Autodesk Inventor part; units mm, degrees
ref_plane "YZ Plane" through (0, 0, 0) normal (1, 0, 0) x (0, 1, 0)
ref_plane "XZ Plane" through (0, 0, 0) normal (0, 1, 0) x (-1, 0, 0)
ref_plane "XY Plane" through (0, 0, 0) normal (0, 0, 1) x (1, 0, 0)
sketch "Sketch1" plane through (0, 0, 0) normal (0, 0, 1) x (1, 0, 0)
  line L0 (-15.5, -9) -> (15.5, -9)
  line L1 (15.5, -9) -> (15.5, 9)
  line L2 (15.5, 9) -> (-15.5, 9)
  line L3 (-15.5, 9) -> (-15.5, -9)
  line L4 (-15.5, -9) -> (15.5, 9) construction
  line L5 (15.5, -9) -> (-15.5, 9) construction
  point P0 (0, 0)
  dimension "d0" = 31
  dimension "d1" = 18
extrude "Extrusion1" add sketch "Sketch1" along normal blind 12.5
sketch "Sketch4" plane through (-15.5, -9, 0) normal (0, -1, 0) x (1, 0, 0)
  line L0 (0, 12.5) -> (31, 12.5)
  circle A0 centre (15.5, 12.5) radius 7.5
  point P0 (15.5, 0)
  dimension "d24" = 15
extrude "Extrusion4" cut sketch "Sketch4" against normal through all
sketch "Sketch5" plane through (0, 0, 12.5) normal (0, 0, 1) x (1, 0, 0)
  line L0 (-15.5, -9) -> (-7.5, -9)
  line L1 (7.5, -9) -> (15.5, -9)
  point P0 (0, 0)
  point P1 (-11.5, 0)
  point P2 (11.5, 0)
  dimension "d86" = 11.5
  dimension "d87" = 11.5
  dimension "d88" = 9
  dimension "d89" = 9
sketch "Sketch8" plane through (-15.5, 9, 0) normal (0, 1, 0) x (1, 0, 0)
  circle A0 centre (6.1, -9.5) radius 1.5
  line L0 (8, -12.5) -> (0, -12.5)
  line L1 (0, 0) -> (0, -12.5)
  point P0 (15.5, 0)
  dimension "d57" = 3
  dimension "d59" = 3
  dimension "d61" = 6.1
hole "Hole1" at (-11.5, 0, 12.5) at (11.5, 0, 12.5) direction (0, 0, -1) diameter 4.3 end through all
extrude "Extrusion11" cut sketch "Sketch8" against normal blind 5.2
sketch "Sketch13" plane through (-15.5, -9, 0) normal (0, -1, 0) x (1, 0, 0)
  arc A0 (8, 12.5) -> (23, 12.5) centre (15.5, 12.5) ccw
  circle A1 centre (15.5, 12.5) radius 8.5
  point P0 (15.5, 0)
  dimension "d99" = 17
extrude "Extrusion12" cut sketch "Sketch13" against normal blind 9
properties part number "Colimador inferior"
Source: CAD feature listing. Evaluate the final solid. Frame: model axes, mm. A direction names the side the tool comes from. Round coordinates to 2 decimals unless told otherwise and drop trailing zeros. Loops run counter-clockwise (first coordinate to the right, second up) from the corner with the lowest first, then second, coordinate; pieces in that order, holes last. Notation, with made-up numbers: M 4,-32.5 L 43,-32.5 A19 ccw 43,-11.5 Z; hole C 61.5,45 d8. An arc over 180 degrees is marked long. Return JSON: item names as keys, results as strings. Group by question number.
1. Pin query (flat end, axial travel): pin 1 (1.5 mm diameter, centred on x = -9, z = 9.5, fed in from +Y). Return the tip coordinate at first contact, or that it passes through.
2. Reachability of faces 1 (the face through (-8.71, 6.44, 10.83)), 2 (the face through (0, -5, 4)), 3 (the face through (10.56, 2.13, 12.5)) from +Z, -Z, +X, -X, +Y, -Y: full face, straight path, thin tool, end or side. Return the list, or none.
3. Section query B-B on y = 7.5. Output: boundary loops of the cut face in (x, z), and give its area (3 significant figures).
4. Section query D-D on y = -1.25. Output: boundary loops of the cut face in (x, z), and give its area (3 significant figures).
5. Material intervals for line 1 along X through (y, z) = (0, 3); line 2 along X through (y, z) = (1.75, 1.25); line 3 along Y through (x, z) = (-11.5, 7.75), sorted ascending. Write a range as from..to.
6. Section query A-A on x = 11.5. Output: boundary loops of the cut face in (y, z), and give its area (3 significant figures).
7. Section query C-C on z = 6. Output: boundary loops of the cut face in (x, y).
8. Mould query, pull axis Y, two halves, no side actions, for faces 4 (the face through (0.6, 0, 4.8)), 5 (the face through (11.41, 2.15, 6.16)), 6 (the face through (-10.192, 1.706, 6.162)), 7 (the face through (-15.5, 0, 6)). Classes: released by +Y, released by -Y, zero draft, split by the parting line, or undercut.
Checks:
{
 "1": {"pin 1": "stops at y = 3.8"},
 "2": {"face 1": "+Y", "face 2": "+Z, -Y", "face 3": "+Z, +X, -X, +Y, -Y"},
 "3": {"outline": "M -15.5,0 L 15.5,0 L 15.5,12.5 L 7.5,12.5 A7.5 cw -7.5,12.5 L -15.5,12.5 Z; hole C -9.4,9.5 d3", "area": "292 mm²"},
 "4": {"outline": "M -15.5,0 L -13.25,0 L -13.25,12.5 L -15.5,12.5 Z; M -9.75,0 L 9.75,0 L 9.75,12.5 L 8.5,12.5 A8.5 cw -8.5,12.5 L -9.75,12.5 Z; M 13.25,0 L 15.5,0 L 15.5,12.5 L 13.25,12.5 Z", "area": "187 mm²"},
 "5": {"line 1": "x = -15.5..-13.65, -9.35..9.35, 13.65..15.5", "line 2": "x = -15.5..-12.75, -10.25..10.25, 12.75..15.5", "line 3": "y = -9..-2.15, 2.15..9"},
 "6": {"outline": "M -9,0 L -2.15,0 L -2.15,12.5 L -9,12.5 Z; M 2.15,0 L 9,0 L 9,12.5 L 2.15,12.5 Z", "area": "171 mm²"},
 "7": {"outline": "M -15.5,-9 L -5.48,-9 L -5.48,0 L -3.74,0 L -3.74,9 L -15.5,9 Z; M 3.74,0 L 5.48,0 L 5.48,-9 L 15.5,-9 L 15.5,9 L 3.74,9 Z; hole C -11.5,0 d4.3; hole C 11.5,0 d4.3"},
 "8": {"face 4": "released by -Y", "face 5": "undercut", "face 6": "undercut", "face 7": "zero draft"}
}
